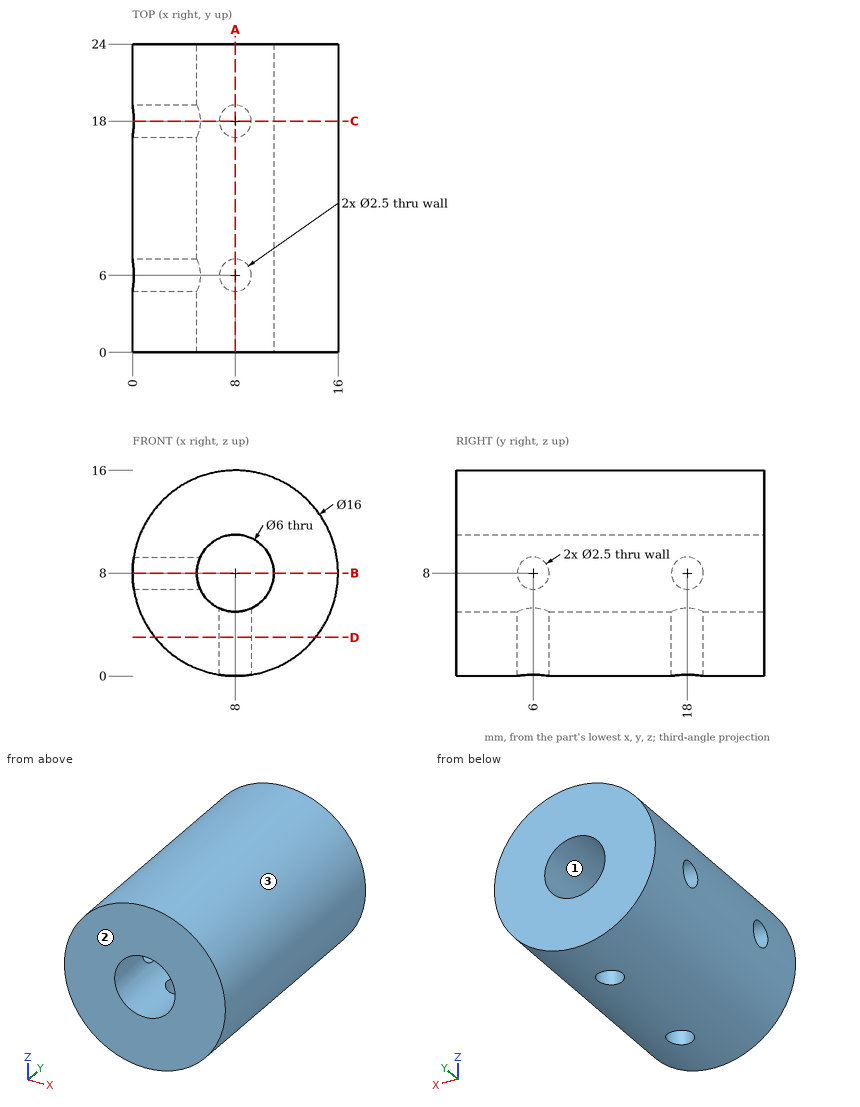
Job drawing, mm, ordinate dimensions from the low corner. One solid piece. Coordinates: 2 decimals unless noted, no trailing zeros. Loops run counter-clockwise (first coordinate to the right, second up) from the corner with the lowest first, then second, coordinate; pieces in that order, holes last. Notation, with made-up numbers: (69, 81) -> (104, 81) arc R8 ccw to (104, 89) -> close; hole circle Ø5 at (86.25, 32). An arc over 180 degrees is marked (long way). One line per item, written item: value.
1. Slice it at B-B on z = 8. Write the cut outline in (x, y).
Answers:
outline: (0, 0) -> (5, 0) -> (5, 4.75) -> (0, 4.75) -> close; (0, 7.25) -> (5, 7.25) -> (5, 16.75) -> (0, 16.75) -> close; (0, 19.25) -> (5, 19.25) -> (5, 24) -> (0, 24) -> close; (11, 0) -> (16, 0) -> (16, 24) -> (11, 24) -> close
2. Flat gauge pins, fed straight in: P1, Ø8, axis at y = 15, z = 14, coming from the +X side; P2, Ø4, axis at x = 3, y = 17, coming from the -Z side; P3, Ø3, axis at x = 11, y = 17, coming from the +Z side. Where does each tip first touch, or does it go through?
Answers:
P1: stops at x = 15.75
P2: stops at z = 0.58
P3: stops at z = 15.86
3. Pull direction Z, two halves, no side cores. Call the marked faces 1, 2 and 3: pulls with the +Z half, pulls with the -Z half, needs draft (parallel to the pull), parting line crosses it, or undercut.
Answers:
face 1: undercut
face 2: needs draft
face 3: parting line crosses it
4. Slice it at C-C on y = 18. Write the cut outline in (x, z), and give its area (3 significant figures).
Answers:
outline: (0.1, 6.75) arc R8 ccw to (6.75, 0.1) -> (6.75, 5.27) arc R3 cw to (5.27, 6.75) -> close; (0.1, 9.25) -> (5.27, 9.25) arc R3 cw (long way) to (9.25, 5.27) -> (9.25, 0.1) arc R8 ccw (long way) to start
area: 148 mm^2
5. Slice it at A-A on x = 8. Write the cut outline in (y, z).
Answers:
outline: (0, 0) -> (4.75, 0) -> (4.75, 5) -> (0, 5) -> close; (0, 11) -> (24, 11) -> (24, 16) -> (0, 16) -> close; (7.25, 0) -> (16.75, 0) -> (16.75, 5) -> (7.25, 5) -> close; (19.25, 0) -> (24, 0) -> (24, 5) -> (19.25, 5) -> close
6. Drill centre lines: line 1 (Y direction, x = 8, z = 1.3); line 2 (Y direction, x = 1.75, z = 9); line 3 (Z direction, x = 8, y = 15). Where is each one in solid material? Low to high. Write a range as [from, to].
Answers:
line 1: y = [0, 4.75], [7.25, 16.75], [19.25, 24]
line 2: y = [0, 5.25], [6.75, 17.25], [18.75, 24]
line 3: z = [0, 5], [11, 16]
7. Slice it at D-D on z = 3. Write the cut outline in (x, y) (3 decimals), and give its area (3 significant figures).
Answers:
outline: (1.755, 0) -> (14.245, 0) -> (14.245, 24) -> (1.755, 24) -> close; hole circle Ø2.5 at (8, 6); hole circle Ø2.5 at (8, 18)
area: 290 mm^2
